Part model, mm, in its own coordinate system. Face numbers are marked on the shaded views. Round coordinates to 2 decimals unless told otherwise and drop trailing zeros. Order: outer loops, then holes, each group sorted by start corner. A loop starts at its lowest first (then second) coordinate and runs counter-clockwise, first axis right, second up. Notation, with made-up numbers: (83, 2.25) - (113, 2.25) arc R19 cw to (113, 11.25) - close; hole circle Ø2 at (25, 19.5). An arc over 180 degrees is marked (long way). Answer as a JSON object with one key per item and string values.
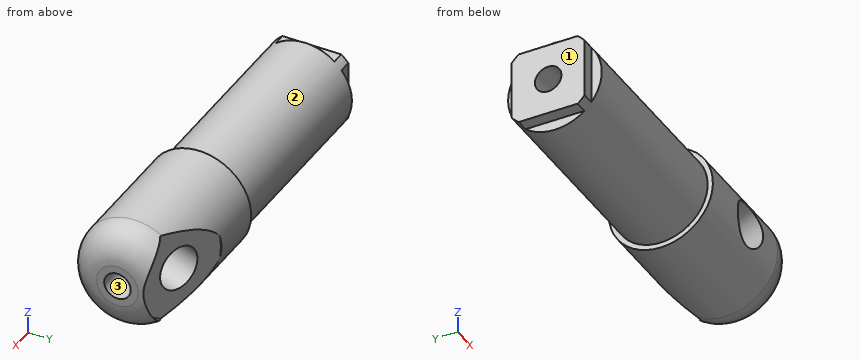
```python
from build123d import *

# Parameters (mm, degrees)
SKETCH1_R               = 10
BOSS_EXTRUDE1_DEPTH     = 69
SKETCH9_OUTSIDE_W       = 36.914
SKETCH9_OUTSIDE_H       = 36.914
SKETCH9_OUTSIDE_R       = 9
CUT_EXTRUDE5_DEPTH      = 40
SKETCH2_OUTSIDE_W       = 36.914
SKETCH2_OUTSIDE_H       = 36.914
SKETCH2_OUTSIDE_W_2     = 14
SKETCH2_OUTSIDE_H_2     = 14
CUT_EXTRUDE1_DEPTH      = 2.4
F_1_4_20_TAPPED_HOLE1_D = 5.1054
FILLET2_R               = 6
SKETCH7_R               = 4.2164
CUT_EXTRUDE2_DEPTH      = 14.501167928
CUT_EXTRUDE2_DEPTH_BACK = 29.892074377
CUT_EXTRUDE3_START      = 7
SKETCH8_R               = 9.525
CUT_EXTRUDE3_DEPTH      = 7.501168056


with BuildPart() as part:
    # Sketch1 → Boss-Extrude1 (new body)
    with BuildSketch(Plane(origin=(0, 0, 0), x_dir=(0, 0, -1), z_dir=(1, 0, 0))):
        Circle(SKETCH1_R)
    extrude(amount=BOSS_EXTRUDE1_DEPTH)

    # Sketch9 outside → Cut-Extrude5 (cut)
    with BuildSketch(Plane.ZY):
        Rectangle(SKETCH9_OUTSIDE_W, SKETCH9_OUTSIDE_H)
        Circle(SKETCH9_OUTSIDE_R, mode=Mode.SUBTRACT)
    extrude(amount=-CUT_EXTRUDE5_DEPTH, mode=Mode.SUBTRACT)

    # Sketch2 outside → Cut-Extrude1 (cut)
    with BuildSketch(Plane.ZY):
        Rectangle(SKETCH2_OUTSIDE_W, SKETCH2_OUTSIDE_H)
        Rectangle(SKETCH2_OUTSIDE_W_2, SKETCH2_OUTSIDE_H_2, mode=Mode.SUBTRACT)
    extrude(amount=-CUT_EXTRUDE1_DEPTH, mode=Mode.SUBTRACT)

    # 1_4-20 Tapped Hole1 (through all)
    with Locations(Plane.ZY):
        with Locations((0, 0)):
            Hole(F_1_4_20_TAPPED_HOLE1_D / 2)

    # Fillet2
    fillet2_edges = [part.edges().sort_by_distance(p)[0] for p in [
        (69, 0, 10),
    ]]
    fillet(fillet2_edges, radius=FILLET2_R)

    # Sketch7 → Cut-Extrude2 (cut, two sides)
    with BuildSketch(Plane(origin=(57, 0, 0), x_dir=(0.939692621, -0.342020143, 0), z_dir=(0.342020143, 0.939692621, 0))) as cut_extrude2_sk:
        Circle(SKETCH7_R)
    extrude(amount=CUT_EXTRUDE2_DEPTH, mode=Mode.SUBTRACT)
    extrude(cut_extrude2_sk.sketch, amount=-CUT_EXTRUDE2_DEPTH_BACK, mode=Mode.SUBTRACT)

    # Sketch8 → Cut-Extrude3 (cut, through all)
    with BuildSketch(Plane(origin=(57, 0, 0), x_dir=(0.939692621, -0.342020143, 0), z_dir=(0.342020143, 0.939692621, 0)).offset(CUT_EXTRUDE3_START)):
        Circle(SKETCH8_R)
    extrude(amount=CUT_EXTRUDE3_DEPTH, mode=Mode.SUBTRACT)


solid = part.part
```
Item 1: Cut at C-C (x = 31). Write the cut outline in (y, z), plus the area to 3 significant figures.
Taken from the geometry:
{"outline": "circle Ø18 at (0, 0); hole circle Ø5.11 at (0, 0)", "area": "234 mm2"}
Item 2: Drop flat-ended pins along their axis: P1, Ø2.5, axis at x = 1, y = 1, coming from the +Z side; P2, Ø1.6, axis at y = 1.5, z = -8, coming from the -X side; P3, Ø10, axis at y = 7, z = 7, coming from the +X side; P4, Ø3, axis at y = 0, z = 0, coming from the +X side. Give the stop position or say it passes through.
Taken from the geometry:
{"P1": "z = 7", "P2": "x = 2.4", "P3": "x = 68.93", "P4": "through"}
Item 3: Cut at A-A (x = 42.5). Write the cut outline in (y, z).
Taken from the geometry:
{"outline": "circle Ø20 at (0, 0); hole circle Ø5.11 at (0, 0)"}
Item 4: Two-plate mould, pull along Z, no slides. Class the marked faces 1, 2 and 3: pulls with the +Z half, pulls with the -Z half, needs draft (parallel to the pull), parting line crosses it, or undercut.
Taken from the geometry:
{"face 1": "needs draft", "face 2": "parting line crosses it", "face 3": "undercut"}
Item 5: Cut at B-B (z = 0). State how many separate pieces and enclosed holes the cut face has, plus the area to 3 significant figures.
Taken from the geometry:
{"separate pieces": "4", "enclosed holes": "0", "area": "762 mm2"}
Item 6: Probe L1, parallel to Z at x = 9, y = -0.25; L2, parallel to Z at x = 33, y = 0; L3, parallel to X at y = -5.25, z = -3.5. List the from-to ranges inside material, lowest first. Write a range as from..to.
Taken from the geometry:
{"L1": "-9..-2.54, 2.54..9", "L2": "-9..-2.55, 2.55..9", "L3": "0..52.59, 57.59..68.54"}
